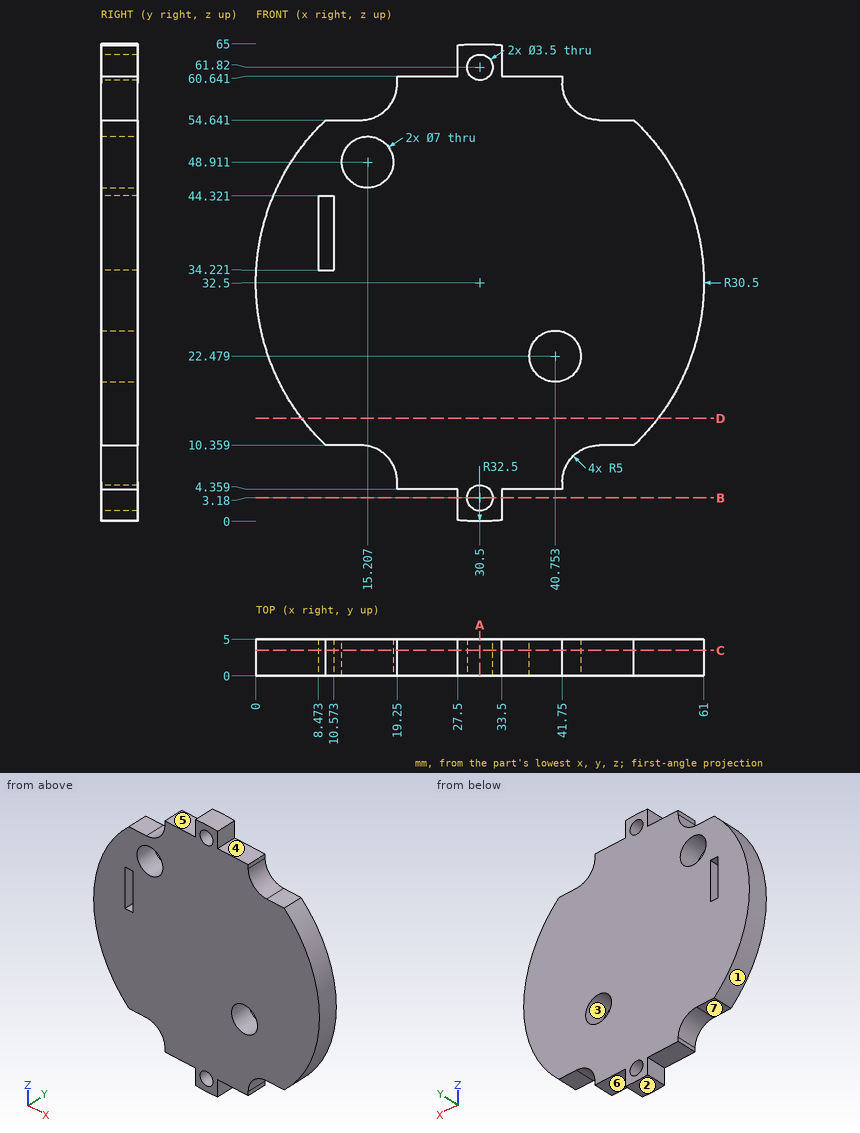
For this review, use the dimensioned drawing (mm, ordinates from the lowest corner) and the shaded views. A direction names the side the tool comes from. Give positions to 0.01 mm unless a question says otherwise; leave off trailing zeros. Loops run counter-clockwise (first coordinate to the right, second up) from the corner with the lowest first, then second, coordinate; pieces in that order, holes last. Notation, with made-up numbers: (12, 52) - (37, 52) arc R23 cw to (37, 85) - close; hole circle Ø6 at (-1.75, 44.25). An arc over 180 degrees is marked (long way). Write each question's results on one line, items separated by ' | '.
(1) Take a section at B-B (z = 3.18). Give the boundary of the cut face in (x, y).
Conclusion:
outline: (27.5, 0) - (28.75, 0) - (28.75, 5) - (27.5, 5) - close; (32.25, 0) - (33.5, 0) - (33.5, 5) - (32.25, 5) - close
(2) Take a section at C-C (y = 3.5). State how many separate pieces and enclosed holes the cut face has, then the cut area to 3 significant figures.
Conclusion:
separate pieces: 1 | enclosed holes: 5 | area: 2,670 mm^2
(3) Take a section at A-A (x = 30.5). Give the boundary of the cut face in (y, z), then the cut area to 3 significant figures.
Conclusion:
outline: (0, 0) - (5, 0) - (5, 1.43) - (0, 1.43) - close; (0, 4.93) - (5, 4.93) - (5, 60.07) - (0, 60.07) - close; (0, 63.57) - (5, 63.57) - (5, 65) - (0, 65) - close | area: 290 mm^2
(4) For line 1 along Z through (x, y) = (30.5, 2.45); line 2 along X through (y, z) = (1.8, 3.18); line 3 along Z through (x, y) = (39.5, 1.4) (1 decimal), list the stretches that pass through material, from the lowest coordinate up.
Conclusion:
line 1: 0 to 1.43, 4.93 to 60.07, 63.57 to 65 | line 2: 27.5 to 28.75, 32.25 to 33.5 | line 3: 4.4 to 19.2, 25.7 to 60.6
(5) For the marked faces 4, 5, 6 and 7, list the 3-axis set-ups (+Z, -Z, +X, -X, +Y, -Y) from which the entire face can be reached by the end or side of a thin tool; tool diameter is ignored.
Conclusion:
face 4: +Z, +X, +Y, -Y | face 5: +Z, -X, +Y, -Y | face 6: -Z, +X, +Y, -Y | face 7: -Z, -X, +Y, -Y
(6) Take a section at D-D (z = 14). Give the boundary of the cut face in (x, y).
Conclusion:
outline: (6.25, 0) - (54.75, 0) - (54.75, 5) - (6.25, 5) - close
(7) For pin 1 Ø2.5 at (y, z) = (2, 37.5) entering from -X; pin 2 Ø0.8 at (y, z) = (2.5, 60) entering from +X; pin 3 Ø1.1 at (y, z) = (2.5, 4.5) entering from -X; pin 4 Ø9 at (x, z) = (40.75, 22.48) entering from +Y, all flat-tipped, find the tip position at first contact; note any pin that passes through.
Conclusion:
pin 1: x = 0.23 | pin 2: x = 41.75 | pin 3: x = 19.25 | pin 4: y = 5
(8) Draft analysis for pull direction X (two halves, no side actions). For the marked faces 1, 2 and 3, state which applies: +X half, -X half, draft (parallel to the pull), parting line (faces both ways), or undercut.
Conclusion:
face 1: -X half | face 2: parting line | face 3: undercut
